from build123d import *

# Parameters (mm, degrees)
F0_W      = 74
F0_H      = 32
F1_DEPTH  = 3
F2_W      = 36.8
F2_H      = 19.2
F3_DEPTH  = 3
F4_R      = 1
F5_R      = 2
F6_DEPTH  = 25
F7_W      = 9
F7_H      = 1.5
F8_DEPTH  = 5
F9_W      = 74
F9_H      = 2
F10_DEPTH = 60
F11_W     = 74
F11_H     = 32
F12_DEPTH = 3
F13_W     = 9
F13_H     = 1.5
F14_DEPTH = 5


with BuildPart() as f1:
    # F0 (on Top) → F1 (new body)
    with BuildSketch(Plane.XY):
        Rectangle(F0_W, F0_H)
    extrude(amount=F1_DEPTH)

    # F2 (on face) → F3 (cut, through all)
    with BuildSketch(Plane.XY.offset(3)):
        with Locations((-3.5, 0.6)):
            Rectangle(F2_W, F2_H)
    extrude(amount=-F3_DEPTH, mode=Mode.SUBTRACT)

    # F4
    f4_edges = [f1.edges().sort_by_distance(p)[0] for p in [
        (-21.9, 10.2, 1.5),
        (-21.9, -9, 1.5),
        (14.9, 10.2, 1.5),
        (14.9, -9, 1.5),
    ]]
    fillet(f4_edges, radius=F4_R)

    # F5 (on face) → F6 (cut)
    with BuildSketch(Plane.XY.offset(3)):
        with Locations((-26.5, 0.6)):
            Circle(F5_R)
        with Locations((25.9, 0.6)):
            Circle(F5_R)
    extrude(amount=-F6_DEPTH, mode=Mode.SUBTRACT)

    # F7 (on face) → F8 (join)
    with BuildSketch(Plane(origin=(0, 16, 0), x_dir=(-1, 0, 0), z_dir=(0, 1, 0))):
        with Locations((0, 1.305378)):
            Rectangle(F7_W, F7_H)
    extrude(amount=F8_DEPTH)

    # F9 (on face) → F10 (join)
    with BuildSketch(Plane(origin=(0, 0, 0), x_dir=(1, 0, 0), z_dir=(0, 0, -1))):
        with Locations((0, 15)):
            Rectangle(F9_W, F9_H)
    extrude(amount=F10_DEPTH)

    # F11 (on face) → F12 (join)
    with BuildSketch(Plane(origin=(0, 0, -60), x_dir=(1, 0, 0), z_dir=(0, 0, -1))):
        Rectangle(F11_W, F11_H)
    extrude(amount=F12_DEPTH)

    # F13 (on face) → F14 (join)
    with BuildSketch(Plane(origin=(0, 16, 0), x_dir=(-1, 0, 0), z_dir=(0, 1, 0))):
        with Locations((0, -63)):
            Rectangle(F13_W, F13_H)
    extrude(amount=F14_DEPTH)


solid = f1.part
Read the model definition and answer for the solid it produces. Units are mm, in the model's axes. A direction names the side the tool comes from. Give positions to 0.01 mm unless a question says otherwise; leave off trailing zeros. Loops run counter-clockwise (first coordinate to the right, second up) from the corner with the lowest first, then second, coordinate; pieces in that order, holes last. Notation, with made-up numbers: (5.5, 8.5) -> (22.5, 8.5) arc R25 cw to (22.5, 23.5) -> close; hole circle Ø1 at (-12.75, 50). An arc over 180 degrees is marked (long way). Use a Markdown table: item, result.
Q1. A tool of negligible diameter and unlimited length cuts with its end or side. For faces 5 (the face through (0, 18, 0.555)), 6 (the face through (-21.9, 0, 2)), 7 (the face through (-37, -14.15, -29.85)), from which of +Z, -Z, +X, -X, +Y, -Y can it reach the whole face along a straight path? Write none if from no direction.
Solved:
| item | result |
|---|---|
| face 5 | +X, -X, +Y |
| face 6 | +Z |
| face 7 | +Z, -Z, -X, +Y, -Y |
Q2. Each of these flat-tipped pins is pushed along its axis until it touches: pin 1 (5 mm diameter, centred on x = -26.5, y = 0.6, fed in from -Z); pin 2 (1.5 mm diameter, centred on x = -16.5, z = -37, fed in from +Y); pin 3 (2.5 mm diameter, centred on x = 25.9, y = 0.6, fed in from +Z). Where does it stop, or does it pass through?
Solved:
| item | result |
|---|---|
| pin 1 | stops at z = -63 |
| pin 2 | stops at y = -14 |
| pin 3 | stops at z = -60 |
Q3. Section B-B, the plane y = 4.5 is taken. Determine the outline of the cut face in (x, z), then the cut area to 3 significant figures.
Solved:
| item | result |
|---|---|
| outline | (-37, -63) -> (37, -63) -> (37, -60) -> (-37, -60) -> close; (-37, 0) -> (-21.9, 0) -> (-21.9, 3) -> (-37, 3) -> close; (14.9, 0) -> (37, 0) -> (37, 3) -> (14.9, 3) -> close |
| area | 334 mm^2 |
Q4. Section C-C, the plane y = 0.6 is taken. Determine the outline of the cut face in (x, z), then the cut area to 3 significant figures.
Solved:
| item | result |
|---|---|
| outline | (-37, -63) -> (37, -63) -> (37, -60) -> (-37, -60) -> close; (-37, 0) -> (-28.5, 0) -> (-28.5, 3) -> (-37, 3) -> close; (-24.5, 0) -> (-21.9, 0) -> (-21.9, 3) -> (-24.5, 3) -> close; (14.9, 0) -> (23.9, 0) -> (23.9, 3) -> (14.9, 3) -> close; (27.9, 0) -> (37, 0) -> (37, 3) -> (27.9, 3) -> close |
| area | 310 mm^2 |
Q5. Determine the mould class of faces 1 (the face through (-1, 11, 0)), 2 (the face through (-4, 10.2, 2)), 3 (the face through (14.9, 0, 2)), 4 (the face through (-1, -14, -30)) for opening direction Y: pulls with the +Y half, pulls with the -Y half, needs draft (parallel to the pull), parting line crosses it, or undercut.
Solved:
| item | result |
|---|---|
| face 1 | needs draft |
| face 2 | undercut |
| face 3 | undercut |
| face 4 | pulls with the +Y half |
Q6. Section D-D, the plane x = 21 is taken. Determine the outline of the cut face in (y, z), then the cut area to 3 significant figures.
Solved:
| item | result |
|---|---|
| outline | (-16, -63) -> (16, -63) -> (16, -60) -> (-14, -60) -> (-14, 0) -> (16, 0) -> (16, 3) -> (-16, 3) -> close |
| area | 312 mm^2 |
Q7. Find the intervals of material crossed by line 1 along Z through (x, y) = (-28, 15.5); line 2 along Y through (x, z) = (25.9, 2.45); line 3 along Y through (x, z) = (30.5, -19), in increasing order.
Solved:
| item | result |
|---|---|
| line 1 | z = -63 to -60, 0 to 3 |
| line 2 | y = -16 to -1.4, 2.6 to 16 |
| line 3 | y = -16 to -14 |
Q8. Section A-A, the plane x = -13 is taken. Determine the outline of the cut face in (y, z).
Solved:
| item | result |
|---|---|
| outline | (-16, -63) -> (16, -63) -> (16, -60) -> (-14, -60) -> (-14, 0) -> (-9, 0) -> (-9, 3) -> (-16, 3) -> close; (10.2, 0) -> (16, 0) -> (16, 3) -> (10.2, 3) -> close |
